Input: part model. Units: mm. Frame: model coordinates. Face numbers are marked on the shaded views. A direction names the side the tool comes from. Round coordinates to 2 decimals unless told otherwise and drop trailing zeros. Loops run counter-clockwise (first coordinate to the right, second up) from the corner with the lowest first, then second, coordinate; pieces in that order, holes last. Notation, with made-up numbers: (58, 88.25) -> (113, 88.25) arc R30 ccw to (113, 123.25) -> close; hole circle Ø6 at (73, -11). An arc over 180 degrees is marked (long way). Answer as a JSON object with one key per item and string values. Group by question number.
Item 1: Section query B-B on y = 7.75. Return loops of the section in (x, z).
Item 2: Section query C-C on y = -1.75. Return loops of the section in (x, z).
Item 3: Section query D-D on z = -23.5. Return loops of the section in (x, y).
Item 4: Set-up query: the marked faces 1 and 2. Return all of +Z, -Z, +X, -X, +Y, -Y with unobstructed straight access to the full face (end or side cutting, diameter ignored); none if empty.
Item 5: Material intervals for line 1 (Y direction, x = 0.5, z = 22.5); line 2 (X direction, y = 3.5, z = 0); line 3 (X direction, y = 7, z = 0), sorted ascending. Write a range as [from, to].
Item 6: Section query A-A on x = -31.5. Return loops of the section in (y, z), and give its area (3 significant figures).
Item 7: Pin query (flat end, axial travel): pin 1 (3 mm diameter, centred on y = 3, z = -2, fed in from -X); pin 2 (3 mm diameter, centred on x = 39.5, y = -1.5, fed in from +Z) (3 decimals); pin 3 (1 mm diameter, centred on x = -2.5, y = 6.5, fed in from -Z). Return the tip coordinate at first contact, or that it passes through.
from build123d import *

# Parameters (mm, degrees)
SKIZZE1_R                       = 52.5
SKIZZE1_R_2                     = 7.5
SKIZZE1_R_3                     = 2.55
AUFSATZ_LINEAR_AUSTRAGEN1_DEPTH = 3
SKIZZE1_3_R                     = 7.5
AUFSATZ_LINEAR_AUSTRAGEN2_DEPTH = 10
VERRUNDUNG1_R                   = 10


with BuildPart() as part:
    # Skizze1 → Aufsatz-Linear austragen1 (new body)
    # profile 1 of 6: a face of its own
    with BuildSketch(Plane(origin=(0, 0, 0), x_dir=(1, 0, 0), z_dir=(0, 1, 0))):
        with Locations(Location((0, 0, 0), (0, 0, 270))):
            Circle(SKIZZE1_R)
        Circle(SKIZZE1_R_2, mode=Mode.SUBTRACT)
    # profile 2 of 6: a face of its own
    with BuildSketch(Plane(origin=(0, 0, 0), x_dir=(1, 0, 0), z_dir=(0, 1, 0))):
        Circle(SKIZZE1_R_2)
        Circle(SKIZZE1_R_3, mode=Mode.SUBTRACT)
    # profile 3 of 6: a face of its own
    with BuildSketch(Plane(origin=(0, 0, 0), x_dir=(1, 0, 0), z_dir=(0, 1, 0))):
        with BuildLine():
            Line((2.272895339, 1.156047913), (-0.601535262, 2.47803457))
            ThreePointArc((-0.601535262, 2.47803457), (-1.576163869, -2.004546697), (2.55, 0))
            ThreePointArc((2.55, 0), (2.47975635, 0.594397546), (2.272895339, 1.156047913))
        make_face()
    # profile 4 of 6: a face of its own
    with BuildSketch(Plane(origin=(0, 0, 0), x_dir=(1, 0, 0), z_dir=(0, 1, 0))):
        with BuildLine():
            ThreePointArc((2.272895339, 1.156047913), (1.065492049, 2.316727583), (-0.601535262, 2.47803457))
            Line((-0.601535262, 2.47803457), (2.272895339, 1.156047913))
        make_face()
    # profile 5 of 6: a face of its own
    with BuildSketch(Plane(origin=(0, 0, 0), x_dir=(1, 0, 0), z_dir=(0, 1, 0))):
        with BuildLine():
            Line((2.272895339, 1.156047913), (-0.601535262, 2.47803457))
            ThreePointArc((-0.601535262, 2.47803457), (-1.576163869, -2.004546697), (2.55, 0))
            ThreePointArc((2.55, 0), (2.47975635, 0.594397546), (2.272895339, 1.156047913))
        make_face()
    # profile 6 of 6: a face of its own
    with BuildSketch(Plane(origin=(0, 0, 0), x_dir=(1, 0, 0), z_dir=(0, 1, 0))):
        with BuildLine():
            ThreePointArc((2.272895339, 1.156047913), (1.065492049, 2.316727583), (-0.601535262, 2.47803457))
            Line((-0.601535262, 2.47803457), (2.272895339, 1.156047913))
        make_face()
    extrude(amount=-AUFSATZ_LINEAR_AUSTRAGEN1_DEPTH)

    # Skizze1<3> → Aufsatz-Linear austragen2 (add)
    with BuildSketch(Plane(origin=(0, 0, 0), x_dir=(1, 0, 0), z_dir=(0, 1, 0))):
        with Locations(Location((0, 0, 0), (0, 0, 270))):
            Circle(SKIZZE1_3_R)
        with BuildLine():
            Line((-0.601535262, 2.47803457), (2.272895339, 1.156047913))
            ThreePointArc((2.272895339, 1.156047913), (-1.065492049, -2.316727583), (-0.601535262, 2.47803457))
        make_face(mode=Mode.SUBTRACT)
    extrude(amount=AUFSATZ_LINEAR_AUSTRAGEN2_DEPTH)

    # Verrundung1
    verrundung1_edges = [part.edges().sort_by_distance(p)[0] for p in [
        (0, 0, -7.5),
    ]]
    fillet(verrundung1_edges, radius=VERRUNDUNG1_R - 0.0001)  # a hair under: the kernel refuses the full size


solid = part.part
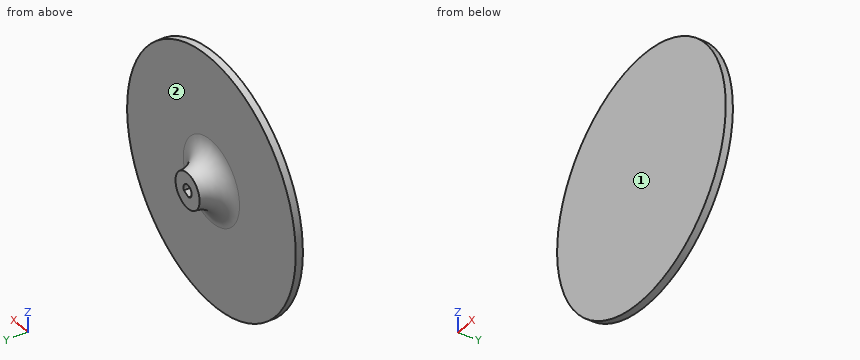
Solved:
{
 "1": {"outline": "circle Ø15.51 at (0, 0); hole (-0.6, -2.48) -> (2.27, -1.16) arc R2.55 ccw (long way) to start"},
 "2": {"outline": "circle Ø105 at (0, 0)"},
 "3": {"outline": "(-46.95, -3) -> (46.95, -3) -> (46.95, 0) -> (-46.95, 0) -> close"},
 "4": {"face 1": "+Z, -Z, +X, -X, -Y", "face 2": "+Y"},
 "5": {"line 1": "[-3, 0]", "line 2": "[-9.9, -2.55], [2.55, 9.9]", "line 3": "[-7.96, -2.55], [2.55, 7.96]"},
 "6": {"outline": "(-3, -42) -> (0, -42) -> (0, 42) -> (-3, 42) -> close", "area": "252 mm²"},
 "7": {"pin 1": "x = -12.08", "pin 2": "z = 36.225", "pin 3": "z = -8"}
}
